Design review of the part built by this model. Coordinates are the model's own, in mm. Face numbers are marked on the shaded views. A direction names the side the tool comes from. Coordinates: 2 decimals unless noted, no trailing zeros. Loops run counter-clockwise (first coordinate to the right, second up) from the corner with the lowest first, then second, coordinate; pieces in that order, holes last. Notation, with made-up numbers: (-26, -31) - (31, -31) arc R20 cw to (31, -12) - close; hole circle Ø5 at (75.25, 59). An arc over 180 degrees is marked (long way). Answer in a Markdown table with one row per item. Add a question column.
(1) We need section C-C, the plane y = 0. Write out the cut boundary in (x, z), plus the area to 3 significant figures.
(2) The part is to be moulded in two halves that separate along X. For the marked faces 4, 5, 6 and 7, say which applies: released by +X, released by -X, zero draft, split by the parting line, or undercut.
(3) We need section D-D, the plane z = 2.9. Write out the cut boundary in (x, y), plus the area to 3 significant figures.
(4) We need section B-B, the plane z = 15. Write out the cut boundary in (x, y).
(5) Clearance check with flat-ended pins moving along their axes: pin 1 (4 mm diameter, centred on y = 27.5, z = 13.5, fed in from -X); pin 2 (2 mm diameter, centred on y = 5, z = 17.5, fed in from +X); pin 3 (6 mm diameter, centred on y = 10, z = 10.5, fed in from +X). State where each tip first meets the part, or that it passes through.
(6) For the marked faces 1, 2 and 3, list the 3-axis set-ups (+Z, -Z, +X, -X, +Y, -Y) from which the entire face can be reached by the end or side of a thin tool; tool diameter is ignored.
(7) We need section A-A, the plane x = 0. Write out the cut boundary in (y, z), plus the area to 3 significant figures.
(8) To check wall thickness, follow L1, parallel to X at y = 16.25, z = 27.1; L2, parallel to Z at x = 0, y = 20; L3, parallel to X at y = 22.75, z = 27.1. State the ranges of each line that lie inside material, in increasing order. Write a range as [from, to].
from build123d import *

# Parameters (mm, degrees)
F1_DEPTH = 30
F2_R     = 1.35
F2_R_2   = 14
F3_DEPTH = 25


with BuildPart() as f1:
    # F0 (on Top) → F1 (new body)
    with BuildSketch(Plane.XY):
        with BuildLine():
            ThreePointArc((-13.462473, -11.797111), (-0.924812, 17.876094), (14.60798, -10.344899))
            Line((14.60798, -10.344899), (16.140658, -11.639981))
            ThreePointArc((16.140658, -11.639981), (19.841413, -1.525887), (17.73066, 9.035137))
            Line((17.73066, 9.035137), (15.409903, 24.723038))
            Line((15.409903, 24.723038), (15.409903, 29.723038))
            Line((15.409903, 29.723038), (-14.590097, 29.723038))
            Line((-14.590097, 29.723038), (-14.590097, 24.723038))
            Line((-14.590097, 24.723038), (-17.73066, 9.035137))
            ThreePointArc((-17.73066, 9.035137), (-19.750704, -2.43304), (-15.007816, -13.068109))
            Line((-15.007816, -13.068109), (-13.462473, -11.797111))
        make_face()
    extrude(amount=F1_DEPTH)

    # F2 (on face) → F3 (cut)
    with BuildSketch(Plane(origin=(0, 29.723038, 0), x_dir=(-1, 0, 0), z_dir=(0, 1, 0))):
        with Locations((-12.509903, 27.1)):
            Circle(F2_R)
        with Locations((-12.509903, 2.9)):
            Circle(F2_R)
        with Locations((11.690097, 2.9)):
            Circle(F2_R)
        with Locations((11.690097, 27.1)):
            Circle(F2_R)
        with Locations((0, 15)):
            Circle(F2_R_2)
    extrude(amount=-F3_DEPTH, mode=Mode.SUBTRACT)


solid = f1.part
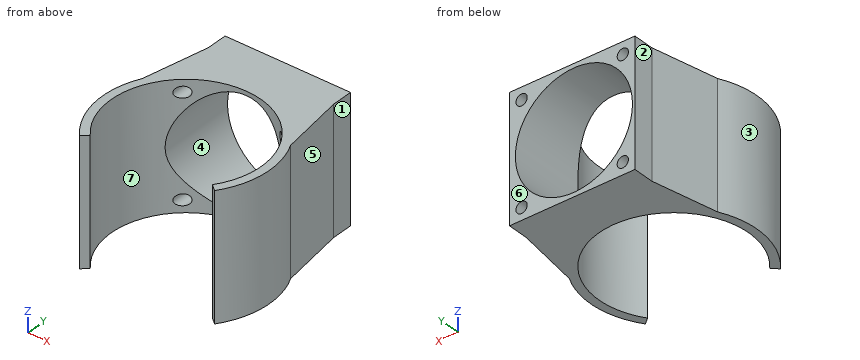
Responses:
| question | item | result |
|---|---|---|
| 1 | outline | (-19.9, 0) - (-17.9, 0) - (-17.9, 30) - (-19.9, 30) - close; (17.9, 0) - (19.9, 0) - (19.9, 30) - (17.9, 30) - close |
| 1 | area | 120 mm2 |
| 2 | face 4 | undercut |
| 2 | face 5 | released by +X |
| 2 | face 6 | zero draft |
| 2 | face 7 | undercut |
| 3 | outline | (-17.73, 9.04) arc R19.9 ccw to (-15.01, -13.07) - (-13.46, -11.8) arc R17.9 cw to (-13.04, 12.26) - (-13.04, 29.72) - (-14.59, 29.72) - (-14.59, 24.72) - close; (-10.34, 14.61) arc R17.9 cw to (-7.04, 16.46) - (-7.04, 29.72) - (-10.34, 29.72) - close; (7.04, 16.46) arc R17.9 cw to (11.16, 14) - (11.16, 29.72) - (7.04, 29.72) - close; (13.86, 11.33) arc R17.9 cw to (14.61, -10.34) - (16.14, -11.64) arc R19.9 ccw to (17.73, 9.04) - (15.41, 24.72) - (15.41, 29.72) - (13.86, 29.72) - close |
| 3 | area | 295 mm2 |
| 4 | outline | (-17.73, 9.04) arc R19.9 ccw to (-15.01, -13.07) - (-13.46, -11.8) arc R17.9 cw to (-14, 11.15) - (-14, 29.72) - (-14.59, 29.72) - (-14.59, 24.72) - close; (14, 11.15) arc R17.9 cw to (14.61, -10.34) - (16.14, -11.64) arc R19.9 ccw to (17.73, 9.04) - (15.41, 24.72) - (15.41, 29.72) - (14, 29.72) - close |
| 5 | pin 1 | stops at x = -14.59 |
| 5 | pin 2 | stops at x = 19.49 |
| 5 | pin 3 | stops at x = 18.63 |
| 6 | face 1 | +Z, -Z, +X, +Y |
| 6 | face 2 | +Z, -Z, -X, +Y |
| 6 | face 3 | +Z, -Z, -X |
| 7 | outline | (17.9, 0) - (29.72, 0) - (29.72, 1) - (17.9, 1) - close; (17.9, 29) - (29.72, 29) - (29.72, 30) - (17.9, 30) - close |
| 7 | area | 23.6 mm2 |
| 8 | L1 | x = [-16.29, -13.04], [-10.34, -7.51], [7.51, 11.16], [13.86, 16.66] |
| 8 | L2 | z = [0, 1], [29, 30] |
| 8 | L3 | x = [-14.99, -13.04], [-10.34, -7.04], [7.04, 11.16], [13.86, 15.7] |
